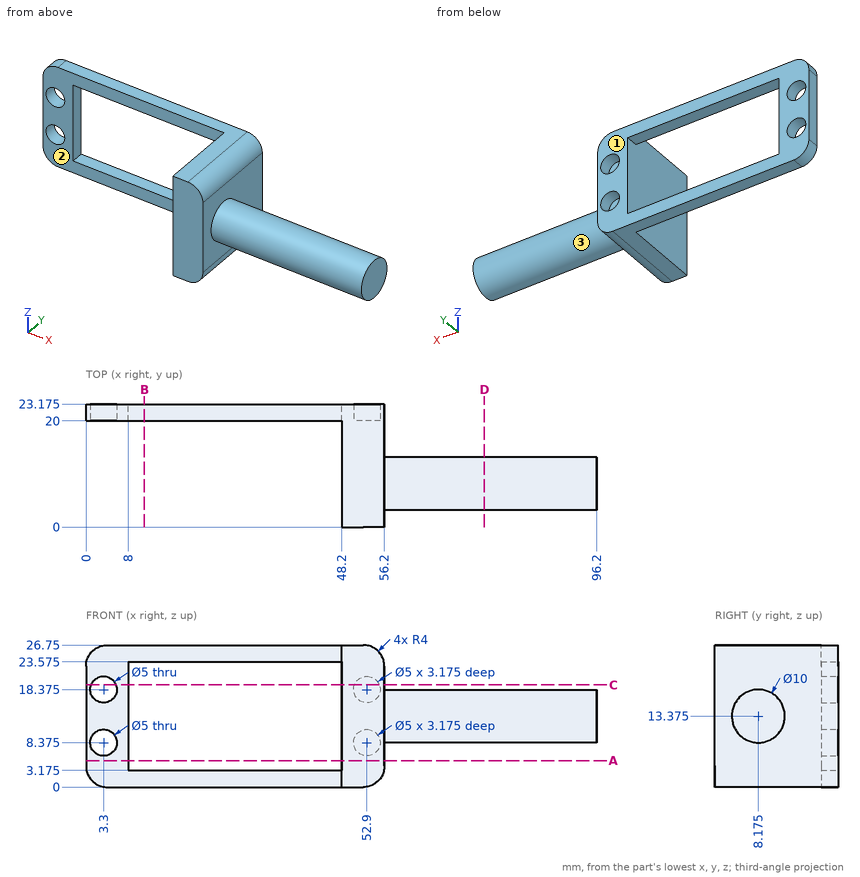
Can you work these out from the drawing? Everything is in mm from the part's minimum corner. A direction names the side the tool comes from. Coordinates: 2 decimals unless noted, no trailing zeros. Loops run counter-clockwise (first coordinate to the right, second up) from the corner with the lowest first, then second, coordinate; pieces in that order, holes last. Notation, with made-up numbers: M -3.75,-25 L 20.25,-25 A26 ccw 20.25,-7 Z; hole C -12.5,9 d2. An arc over 180 degrees is marked long. One line per item, written item: value.
1. Imagine slicing it at A-A (z = 5). List the corners of the cut face in (x, y) for me (3 decimals).
Geometry says:
outline: M 0,20 L 8,20 L 8,23.175 L 0,23.175 Z; M 48.2,0 L 56.2,0 L 56.2,23.175 L 48.2,23.175 Z
2. Will these pins go through, and if not, where does the flat tip stop? pin 1 Ø10 at (y, z) = (20, 6.5) entering from +X; pin 2 Ø4.5 at (x, z) = (3.3, 18.375) entering from +Y; pin 3 Ø6 at (x, z) = (65.5, 15.5) entering from -Y (3 decimals); pin 4 Ø10 at (y, z) = (4, 8) entering from -X.
Geometry says:
pin 1: stops at x = 56.2
pin 2: passes through
pin 3: stops at y = 3.175
pin 4: stops at x = 48.2
3. On a 3-axis mill with a long thin cutter (end or side, diameter ignored), from which of +Z, -Z, +X, -X, +Y, -Y can I reach the whole of each face in a straight line? I mean the marked faces 1, 2 and 3. Say none if no direction works.
Geometry says:
face 1: +Z, -Z, +X, -X, +Y
face 2: +Z, -Z, -X, -Y
face 3: +X
4. Imagine slicing it at D-D (x = 75). List the corners of the cut face in (y, z) for me (3 decimals), and give its area (3 significant figures).
Geometry says:
outline: C 8.175,13.375 d10
area: 78.5 mm2
5. Imagine slicing it at C-C (z = 19.25). List the corners of the cut face in (x, y) for me (3 decimals).
Geometry says:
outline: M 0,20 L 0.958,20 L 0.958,23.175 L 0,23.175 Z; M 5.642,20 L 8,20 L 8,23.175 L 5.642,23.175 Z; M 48.2,0 L 56.2,0 L 56.2,23.175 L 55.242,23.175 L 55.242,20 L 50.558,20 L 50.558,23.175 L 48.2,23.175 Z
6. Please list where these lines run through material, in increasing order: probe 1 along Y at (x, z) = (65.5, 13); probe 2 along X at (y, z) = (5.5, 17.5); probe 3 along X at (y, z) = (19.75, 5.5).
Geometry says:
probe 1: y = 3.19 to 13.16
probe 2: x = 48.2 to 96.2
probe 3: x = 48.2 to 56.2
7. Imagine slicing it at B-B (x = 11). List the corners of the cut face in (y, z) for me (3 decimals).
Geometry says:
outline: M 20,0 L 23.175,0 L 23.175,3.175 L 20,3.175 Z; M 20,23.575 L 23.175,23.575 L 23.175,26.75 L 20,26.75 Z
